```python
from build123d import *

# Parameters (mm, degrees)
F0_W     = 25.4
F0_H     = 25.4
F0_W_2   = 22.098
F0_H_2   = 22.098
F1_DEPTH = 1625.6
F3_DEPTH = 25.401
F5_DEPTH = 25.401


with BuildPart() as f1:
    # F0 (on Front) → F1 (new body)
    with BuildSketch(Plane.XZ):
        with Locations((12.7, 12.7)):
            Rectangle(F0_W, F0_H)
        with Locations((12.7, 12.7)):
            Rectangle(F0_W_2, F0_H_2, mode=Mode.SUBTRACT)
    extrude(amount=F1_DEPTH)

    # F2 (on face) → F3 (cut, through all)
    with BuildSketch(Plane.XY.offset(25.4)):
        Polygon((0, -1625.6), (25.4, -1625.6), (0, -1600.2), align=None)
    extrude(amount=-F3_DEPTH, mode=Mode.SUBTRACT)

    # F4 (on face) → F5 (cut, through all)
    with BuildSketch(Plane.XY.offset(25.4)):
        Polygon((0, -25.4), (25.4, 0), (0, 0), align=None)
    extrude(amount=-F5_DEPTH, mode=Mode.SUBTRACT)


solid = f1.part
```
Verification items for the finished model (mm, model axes). Coordinates: 2 decimals unless noted, no trailing zeros. Write each loop counter-clockwise with the first axis right and the second up, starting at its lowest first coordinate (ties: lowest second). Pieces come first, ordered by that corner, then holes. Notation, with made-up numbers: (53, 80) - (92, 80) arc R16 cw to (92, 95) - close; hole circle Ø11 at (36, 72). An arc over 180 degrees is marked (long way). Write item = value, one per line.
Q1. Cross-section at B-B (y = -186). Enter the section's corners in (x, z).
Answer:
outline = (0, 0) - (25.4, 0) - (25.4, 25.4) - (0, 25.4) - close; hole (1.65, 1.65) - (23.75, 1.65) - (23.75, 23.75) - (1.65, 23.75) - close
Q2. Material ranges on L1, parallel to Z at x = 8.5, y = -168, recorded low to high. Write a range as from..to.
Answer:
L1 = 0..1.65, 23.75..25.4
Q3. Cross-section at C-C (z = 14.75). Enter the section's corners in (x, y).
Answer:
outline = (0, -1600.2) - (1.65, -1601.85) - (1.65, -23.75) - (0, -25.4) - close; (23.75, -1623.95) - (25.4, -1625.6) - (25.4, 0) - (23.75, -1.65) - close
Q4. Cross-section at A-A (x = 17.75). Enter the section's corners in (y, z).
Answer:
outline = (-1617.95, 0) - (-7.65, 0) - (-7.65, 1.65) - (-1617.95, 1.65) - close; (-1617.95, 23.75) - (-7.65, 23.75) - (-7.65, 25.4) - (-1617.95, 25.4) - close
